from build123d import *

# Parameters (mm, degrees)
F1_DEPTH       = 40
F2_T1_DEPTH    = 40
F5_DEPTH       = 40
F6_W           = 23.4
F6_H           = 0.5
F7_DEPTH       = 40.001
F8_T1_DEPTH    = 40
F9_W           = 5
F9_H           = 10
F10_DEPTH      = 181
F10_DEPTH_BACK = 4.501


# Not quite as in the source:
# - a fillet or chamfer that OpenCascade refuses, or shapes differently, is made with other operations: its cross-section is extruded or revolved along the edge and cut away or added
# - an extrude ends at something that could not be found from the text; its depth is read off the source's solid


with BuildPart() as f1:
    # F0 (on Front) → F1 (new body)
    with BuildSketch(Plane.XZ):
        Polygon((77.5, 0), (0, 0), (0, -2), (50.1, -2), (50.1, -4.5), (53.1, -4.5), (53.1, -3.6), (52.1, -3.6), (52.1, -2), (52.1, -1.5), (75.5, -1.5), (75.5, -2), (75.5, -3.6), (74.5, -3.6), (74.5, -4.5), (77.5, -4.5), (77.5, -2), align=None)
    extrude(amount=F1_DEPTH)

    # F2: fillet of radius 5 on 1 edges, made by hand

    # F2_s2 → F2_t1 (join)
    with BuildSketch(Plane.XZ):
        with BuildLine():
            ThreePointArc((50.1, -4.5), (48.2698729811, -2.6698729811), (45.7698729811, -2))
            Line((45.7698729811, -2), (50.1, -2))
            Line((50.1, -2), (50.1, -4.5))
        make_face()
    extrude(amount=F2_T1_DEPTH)

    # F3: F1 across plane


with BuildPart() as f1_1:
    add(f1.part)
    add(f1.part.mirror(Plane.YZ))

    # F4 (on face) → F5 (join, through all)
    with BuildSketch(Plane.XZ.offset(40)):
        Polygon((-17.4, -3.6), (-17.4, -2), (-19.4, -2), (-19.4, -4.5), (-17.4, -4.5), (-16.4, -4.5), (-16.4, -3.6), align=None)
        Polygon((8, -2), (6, -2), (6, -3.6), (5, -3.6), (5, -4.5), (6, -4.5), (8, -4.5), align=None)
    extrude(amount=-F5_DEPTH)

    # F6 (on face) → F7 (cut, through all)
    with BuildSketch(Plane(origin=(0, 0, 0), x_dir=(-1, 0, 0), z_dir=(0, 1, 0))):
        with Locations((5.7, -1.75)):
            Rectangle(F6_W, F6_H)
    extrude(amount=-F7_DEPTH, mode=Mode.SUBTRACT)

    # F8: fillet of radius 5 on 2 edges, made by hand

    # F8_s2 → F8_t1 (join)
    with BuildSketch(Plane.XZ):
        with BuildLine():
            ThreePointArc((-19.4, -4.5), (-21.2301270189, -2.6698729811), (-23.7301270189, -2))
            Line((-23.7301270189, -2), (-19.4, -2))
            Line((-19.4, -2), (-19.4, -4.5))
        make_face()
        with BuildLine():
            ThreePointArc((12.3301270189, -2), (9.8301270189, -2.6698729811), (8, -4.5))
            Line((8, -4.5), (8, -2))
            Line((8, -2), (12.3301270189, -2))
        make_face()
    extrude(amount=F8_T1_DEPTH)

    # F9 (on Top) → F10 (cut, two sides)
    with BuildSketch(Plane.XY) as f10_sk:
        with Locations((-24.5, -35)):
            Rectangle(F9_W, F9_H)
    extrude(amount=F10_DEPTH, mode=Mode.SUBTRACT)
    extrude(f10_sk.sketch, amount=-F10_DEPTH_BACK, mode=Mode.SUBTRACT)


solid = f1_1.part
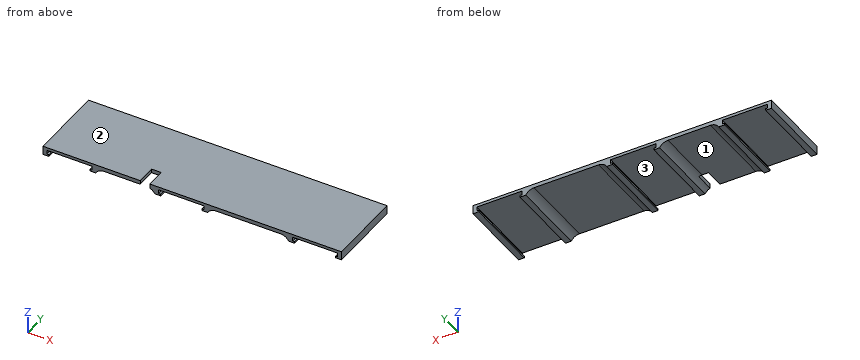
Design review of the part built by this model. Coordinates are the model's own, in mm. Face numbers are marked on the shaded views. Coordinates: 2 decimals unless noted, no trailing zeros. Write each loop counter-clockwise with the first axis right and the second up, starting at its lowest first coordinate (ties: lowest second). Pieces come first, ordered by that corner, then holes. Notation, with made-up numbers: (18, -19.5) - (71, -19.5) arc R19 ccw to (71, -1.5) - close; hole circle Ø7 at (-38, 18). An arc over 180 degrees is marked (long way). One line per item, written item: value.
1) To check wall thickness, follow probe 1 along X at (y, z) = (-37, -1.7); probe 2 along X at (y, z) = (-4, -4.05); probe 3 along X at (y, z) = (-29, -3.35). State the ranges of each line that lie inside material, in increasing order.
Answer sheet:
probe 1: x = -77.5 to -75.5, -52.1 to -27, -22 to -17.4, 6 to 52.1, 75.5 to 77.5
probe 2: x = -77.5 to -74.5, -53.1 to -49.81, -19.69 to -16.4, 5 to 8.29, 49.81 to 53.1, 74.5 to 77.5
probe 3: x = -77.5 to -75.5, -52.1 to -49.19, -20.31 to -17.4, 6 to 8.91, 49.19 to 52.1, 75.5 to 77.5
2) Add section B-B (x = 39.5). State the section outline as (y, z) points.
Answer sheet:
outline: (-40, -2) - (0, -2) - (0, 0) - (-40, 0) - close
3) Add section A-A (x = -8.5). State the section outline as (y, z) points.
Answer sheet:
outline: (-40, -1.5) - (0, -1.5) - (0, 0) - (-40, 0) - close
4) Mouldability with a two-part tool opening along X and no side actions: class the marked faces 1, 2 and 3 as +X half, -X half, draft (parallel to the pull), parting line (faces both ways), or undercut.
Answer sheet:
face 1: undercut
face 2: draft
face 3: undercut
5) Insertion check: pin 1 (11.5 mm diameter, centred on x = -3.5, y = -14, fed in from -Z); pin 2 (24 mm diameter, centred on x = -37.5, y = -15, fed in from -Z); pin 3 (2 mm diameter, centred on x = 33, y = -24, fed in from -Z). Each pin has a flat end and moves straight along its axis. Give the tip position at first contact, or say it passes through.
Answer sheet:
pin 1: stops at z = -1.5
pin 2: stops at z = -3.67
pin 3: stops at z = -2
